Source: CAD feature listing. Evaluate the final solid. Frame: model axes, mm. A direction names the side the tool comes from. Give positions to 0.01 mm unless a question says otherwise; leave off trailing zeros. Write each loop counter-clockwise with the first axis right and the second up, starting at its lowest first coordinate (ties: lowest second). Pieces come first, ordered by that corner, then holes. Notation, with made-up numbers: (5.25, 3.5) -> (12.25, 3.5) arc R22 cw to (12.25, 9.5) -> close; hole circle Ø2 at (-7.75, 82.5). An arc over 180 degrees is marked (long way). Answer as a JSON object with one key per item and string values. Group by question number.
Item 1: Access query for faces 5 (the face through (19, -10, 444)), 6 (the face through (17.44, -10, 444)). Directions: +Z, -Z, +X, -X, +Y, -Y. A direction counts if a zero-diameter tool reaches every point of the face in a straight line with its end or side. Return the directions, or none.
Item 2: Section query A-A on x = 14.5. Return the cut outline in (y, z), plus the area to 3 significant figures.
Item 3: Ray query, probe 1 along Y at (x, z) = (13.75, 353); probe 2 along X at (y, z) = (-13.25, 687.5). Return the intervals inside material, ascending. Write a range as from..to.
Item 4: Pull-direction query (Y, two-part tool) for faces 1 (the face through (9, -19, 444)), 2 (the face through (9, 0, 444)), 3 (the face through (9, -18, 0)), 4 (the face through (9, -17.44, 444)); classes: pulls with the +Y half, pulls with the -Y half, needs draft (parallel to the pull), parting line crosses it, or undercut.
Item 5: Section query B-B on z = 335. Return the cut outline in (x, y), plus the area to 3 significant figures.
Item 6: Section query C-C on y = -5.25. Return the cut outline in (x, z).
Item 7: First-contact query: pin 1 Ø1.5 at (x, y) = (8.5, -16.5) entering from +Z. Flat tip, straight axial feed; report the tip coordinate or a pass-through.
from build123d import *

# Parameters (mm, degrees)
SKETCH_1_W      = 19
SKETCH_1_H      = 19
SKETCH_1_W_2    = 15.88
SKETCH_1_H_2    = 15.88
EXTRUDE_1_DEPTH = 900
FILLET_2_R      = 1


with BuildPart() as part:
    # 스케치1 → 보스-돌출1 (new body)
    with BuildSketch(Plane.XY):
        with Locations((9.5, -9.5)):
            Rectangle(SKETCH_1_W, SKETCH_1_H)
        with Locations((9.5, -9.5)):
            Rectangle(SKETCH_1_W_2, SKETCH_1_H_2, mode=Mode.SUBTRACT)
    extrude(amount=EXTRUDE_1_DEPTH)

    # 필렛2
    fillet_2_edges = [part.edges().sort_by_distance(p)[0] for p in [
        (0, 0, 450),
        (19, 0, 450),
        (19, -19, 450),
        (0, -19, 450),
    ]]
    fillet(fillet_2_edges, radius=FILLET_2_R)


solid = part.part
Worked answers:
{
 "1": {"face 5": "+Z, -Z, +X, +Y, -Y", "face 6": "+Z, -Z"},
 "2": {"outline": "(-19, 0) -> (-17.44, 0) -> (-17.44, 900) -> (-19, 900) -> close; (-1.56, 0) -> (0, 0) -> (0, 900) -> (-1.56, 900) -> close", "area": "2,810 mm^2"},
 "3": {"probe 1": "-19..-17.44, -1.56..0", "probe 2": "0..1.56, 17.44..19"},
 "4": {"face 1": "pulls with the -Y half", "face 2": "pulls with the +Y half", "face 3": "needs draft", "face 4": "undercut"},
 "5": {"outline": "(0, -18) arc R1 ccw to (1, -19) -> (18, -19) arc R1 ccw to (19, -18) -> (19, -1) arc R1 ccw to (18, 0) -> (1, 0) arc R1 ccw to (0, -1) -> close; hole (1.56, -17.44) -> (17.44, -17.44) -> (17.44, -1.56) -> (1.56, -1.56) -> close", "area": "108 mm^2"},
 "6": {"outline": "(0, 0) -> (1.56, 0) -> (1.56, 900) -> (0, 900) -> close; (17.44, 0) -> (19, 0) -> (19, 900) -> (17.44, 900) -> close"},
 "7": {"pin 1": "through"}
}
